Can you work these out from the drawing? Everything is in mm from the part's minimum corner. A direction names the side the tool comes from. Round coordinates to 2 decimals unless told otherwise and drop trailing zeros. Loops run counter-clockwise (first coordinate to the right, second up) from the corner with the lowest first, then second, coordinate; pieces in that order, holes last. Notation, with made-up numbers: (56, 35.5) -> (101, 35.5) arc R17 cw to (101, 51.5) -> close; hole circle Ø5 at (68.5, -5). An arc over 180 degrees is marked (long way). One line per item, written item: value.
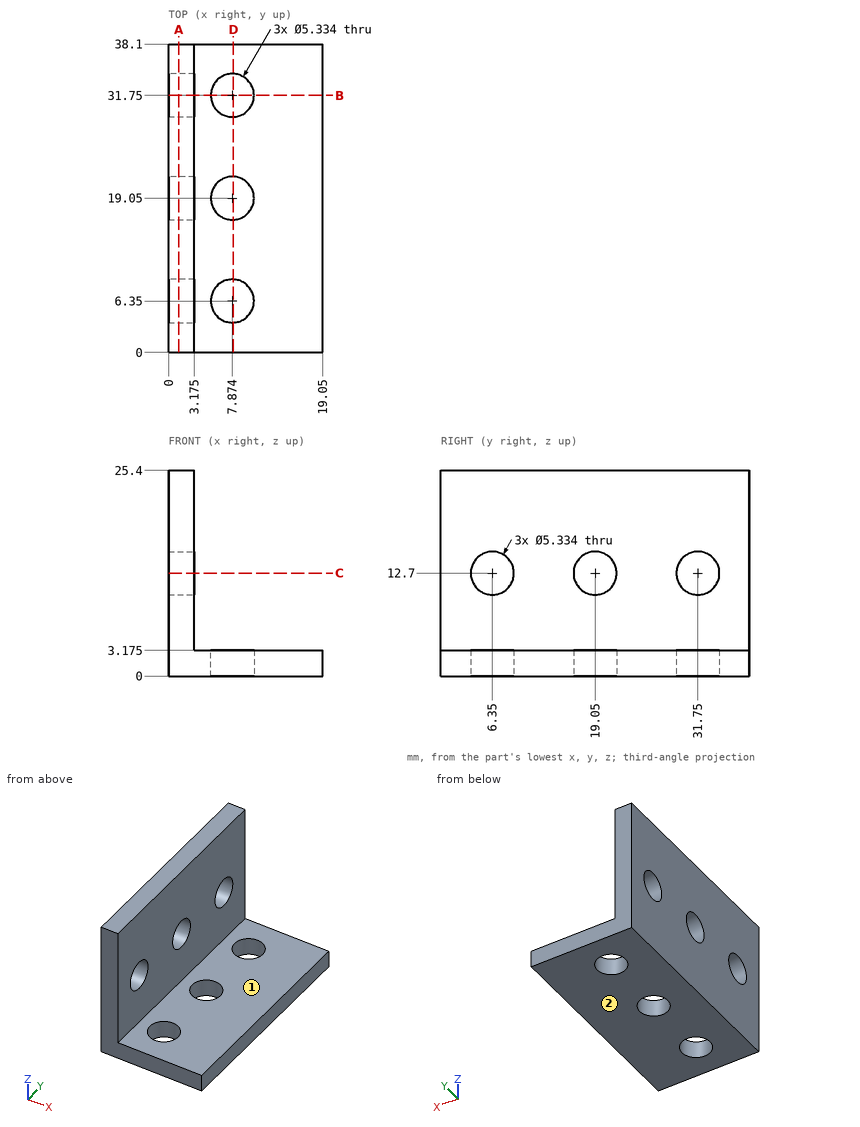
(1) On a 3-axis mill with a long thin cutter (end or side, diameter ignored), from which of +Z, -Z, +X, -X, +Y, -Y can I reach the whole of each face in a straight line? I mean the marked faces 1 and 2. Say none if no direction works.
Results below:
face 1: +Z, +X, +Y, -Y
face 2: -Z, +X, -X, +Y, -Y
(2) For pin 1 Ø10 at (y, z) = (7.5, 20) entering from +X (3 decimals); pin 2 Ø3 at (x, y) = (12.5, 10.5) entering from +Z (3 decimals); pin 3 Ø8.5 at (y, z) = (19.05, 12.7) entering from -X, each with a flat end and sliding along its axis, tell me the tip position at first contact or that it passes through.
Results below:
pin 1: stops at x = 3.175
pin 2: stops at z = 3.175
pin 3: stops at x = 0
(3) Imagine slicing it at B-B on y = 31.75. Write out the boundary of the cut face in (x, z) (3 decimals).
Results below:
outline: (0, 0) -> (5.207, 0) -> (5.207, 3.175) -> (3.175, 3.175) -> (3.175, 10.033) -> (0, 10.033) -> close; (0, 15.367) -> (3.175, 15.367) -> (3.175, 25.4) -> (0, 25.4) -> close; (10.541, 0) -> (19.05, 0) -> (19.05, 3.175) -> (10.541, 3.175) -> close
(4) Please list where these lines run through material, in increasing order: L1, parallel to X at y = 31.75, z = 2.3; L2, parallel to Z at x = 2.25, y = 31.75; L3, parallel to X at y = 19.5, z = 9.5 (3 decimals).
Results below:
L1: x = 0 to 5.21, 10.54 to 19.05
L2: z = 0 to 10.03, 15.37 to 25.4
L3: x = 0 to 3.175
(5) Imagine slicing it at D-D on x = 8. Write out the boundary of the cut face in (y, z) (3 decimals), then the cut area to 3 significant figures.
Results below:
outline: (0, 0) -> (3.686, 0) -> (3.686, 3.175) -> (0, 3.175) -> close; (9.014, 0) -> (16.386, 0) -> (16.386, 3.175) -> (9.014, 3.175) -> close; (21.714, 0) -> (29.086, 0) -> (29.086, 3.175) -> (21.714, 3.175) -> close; (34.414, 0) -> (38.1, 0) -> (38.1, 3.175) -> (34.414, 3.175) -> close
area: 70.2 mm²
(6) Imagine slicing it at C-C on z = 12.7. Write out the boundary of the cut face in (x, y) (3 decimals), then the cut area to 3 significant figures.
Results below:
outline: (0, 0) -> (3.175, 0) -> (3.175, 3.683) -> (0, 3.683) -> close; (0, 9.017) -> (3.175, 9.017) -> (3.175, 16.383) -> (0, 16.383) -> close; (0, 21.717) -> (3.175, 21.717) -> (3.175, 29.083) -> (0, 29.083) -> close; (0, 34.417) -> (3.175, 34.417) -> (3.175, 38.1) -> (0, 38.1) -> close
area: 70.2 mm²
(7) Imagine slicing it at A-A on x = 1.25. Write out the boundary of the cut face in (y, z).
Results below:
outline: (0, 0) -> (38.1, 0) -> (38.1, 25.4) -> (0, 25.4) -> close; hole circle Ø5.33 at (6.35, 12.7); hole circle Ø5.33 at (19.05, 12.7); hole circle Ø5.33 at (31.75, 12.7)
